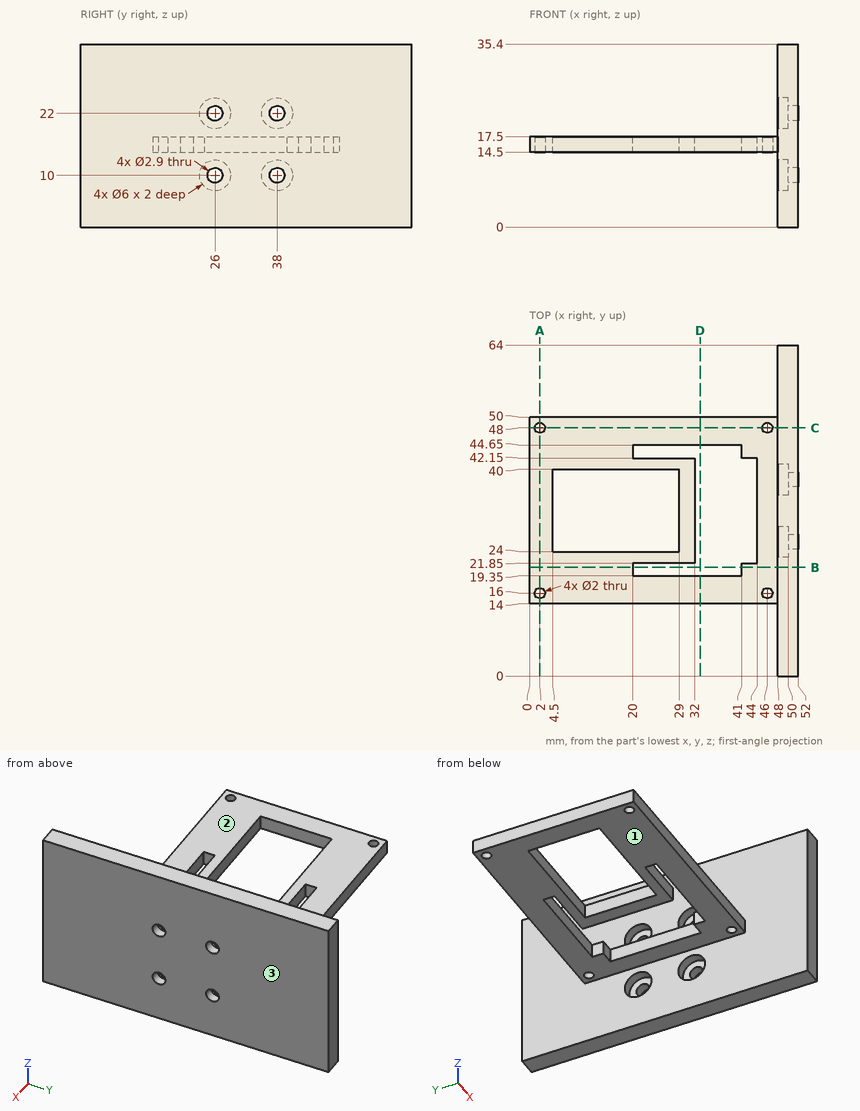
Here's the drawing with two shaded views (mm, measured from the low corner). I have some questions. A direction names the side the tool comes from. Coordinates: 2 decimals unless noted, no trailing zeros. Write each loop counter-clockwise with the first axis right and the second up, starting at its lowest first coordinate (ties: lowest second). Pieces come first, ordered by that corner, then holes. Notation, with made-up numbers: (71.5, 77) -> (103.5, 77) arc R19 ccw to (103.5, 100) -> close; hole circle Ø2 at (86, -24.75). An arc over 180 degrees is marked (long way). Write item = value, one per line. Start each with the question number.
(1) I need wall thicknesses on line 1 (X direction, y = 48, z = 16.85); line 2 (Y direction, x = 51.5, z = 10); line 3 (Y direction, x = 46, z = 15). Which ranges of each line are inside material? Lowest first, please. Write a range as [from, to].
(2) I want a section at C-C (y = 48). Please give me the cut outline in (x, z), plus the area to 3 significant figures.
(3) I want a section at D-D (x = 33). Please give me the cut outline in (y, z).
(4) I want a section at B-B (y = 21). Please give me the cut outline in (x, z), plus the area to 3 significant figures.
(5) Which directions (+Z, -Z, +X, -X, +Y, -Y) give clear straight access to the entire face, cutting with the end or side of a thin tool? Please do the marked faces 1, 2 and 3.
(6) Will these pins go through, and if not, where does the flat tip stop? pin 1 (0.9 mm diameter, centred on x = 34.5, z = 16.5, fed in from -Y); pin 2 (2 mm diameter, centred on y = 43, z = 16, fed in from -X); pin 3 (3.5 mm diameter, centred on x = 28.5, z = 16, fed in from +Y); pin 4 (2 mm diameter, centred on y = 15, z = 4, fed in from -X).
(7) I want a section at A-A (x = 2). Please give me the cut outline in (y, z), plus the area to 3 significant figures.
Result set:
q1.line_1 = [0, 1], [3, 45], [47, 52]
q1.line_2 = [0, 24.55], [27.45, 36.55], [39.45, 64]
q1.line_3 = [14, 15], [17, 47], [49, 50]
q2.outline = (0, 14.5) -> (1, 14.5) -> (1, 17.5) -> (0, 17.5) -> close; (3, 14.5) -> (45, 14.5) -> (45, 17.5) -> (3, 17.5) -> close; (47, 14.5) -> (48, 14.5) -> (48, 0) -> (52, 0) -> (52, 35.4) -> (48, 35.4) -> (48, 17.5) -> (47, 17.5) -> close
q2.area = 274 mm2
q3.outline = (14, 14.5) -> (19.35, 14.5) -> (19.35, 17.5) -> (14, 17.5) -> close; (44.65, 14.5) -> (50, 14.5) -> (50, 17.5) -> (44.65, 17.5) -> close
q4.outline = (0, 14.5) -> (20, 14.5) -> (20, 17.5) -> (0, 17.5) -> close; (41, 14.5) -> (48, 14.5) -> (48, 0) -> (52, 0) -> (52, 35.4) -> (48, 35.4) -> (48, 17.5) -> (41, 17.5) -> close
q4.area = 223 mm2
q5.face_1 = -Z, -X, +Y, -Y
q5.face_2 = +Z, -X, +Y, -Y
q5.face_3 = +Z, -Z, +X, +Y, -Y
q6.pin_1 = 14
q6.pin_2 = 0
q6.pin_3 = 50
q6.pin_4 = 48
q7.outline = (14, 14.5) -> (15, 14.5) -> (15, 17.5) -> (14, 17.5) -> close; (17, 14.5) -> (47, 14.5) -> (47, 17.5) -> (17, 17.5) -> close; (49, 14.5) -> (50, 14.5) -> (50, 17.5) -> (49, 17.5) -> close
q7.area = 96.0 mm2
